```python
from build123d import *

# Parameters (mm, degrees)
SKETCH_1_W          = 55
SKETCH_1_H          = 20
SKETCH_1_R          = 4.5
EXTRUDE_1_DEPTH     = 20
EXTRUDE_START       = -10
EXTRUDE_2_OUTLINE_W = 13.25368731
EXTRUDE_2_OUTLINE_H = 35
EXTRUDE_2_DEPTH     = 20
SKETCH_3_R          = 5.25
CUT_EXTRUDE_1_DEPTH = 30
FILLET1_R           = 10
FILLET2_R           = 3
FILLET3_R           = 3


# Read off the part's stored shape, not the designer's step: 填料-伸長2
with BuildPart() as part:
    # 草圖1 → 填料-伸長1 (new body)
    with BuildSketch(Plane(origin=(0, 0, 0), x_dir=(1, 0, 0), z_dir=(0, 1, 0))):
        Rectangle(SKETCH_1_W, SKETCH_1_H)
        with Locations(Location((-15, 0, 0), (0, 0, 270))):
            Circle(SKETCH_1_R, mode=Mode.SUBTRACT)
        with Locations(Location((15, 0, 0), (0, 0, 90))):
            Circle(SKETCH_1_R, mode=Mode.SUBTRACT)
    extrude(amount=EXTRUDE_1_DEPTH)

    # 填料-伸長2 outline → 填料-伸長2 (add)
    with BuildSketch(Plane.XY.offset(EXTRUDE_START)):
        with Locations((0, 37.5)):
            Rectangle(EXTRUDE_2_OUTLINE_W, EXTRUDE_2_OUTLINE_H)
    extrude(amount=EXTRUDE_2_DEPTH)

    # 草圖3 → 除料-伸長1 (cut)
    with BuildSketch(Plane(origin=(6.626843655, 0, 0), x_dir=(0, 0, -1), z_dir=(1, 0, 0))):
        with Locations((0.362292653, 41.5)):
            Circle(SKETCH_3_R)
    extrude(amount=-CUT_EXTRUDE_1_DEPTH, mode=Mode.SUBTRACT)

    # Fillet1
    fillet1_edges = [part.edges().sort_by_distance(p)[0] for p in [
        (0, 55, -10),
        (0, 55, 10),
    ]]
    fillet(fillet1_edges, radius=FILLET1_R - 0.0001)  # a hair under: the kernel refuses the full size

    # Fillet2
    fillet2_edges = [part.edges().sort_by_distance(p)[0] for p in [
        (-27.5, 20, 0),
        (-17.063421827, 20, 10),
        (-17.063421827, 20, -10),
    ]]
    fillet(fillet2_edges, radius=FILLET2_R)

    # Fillet3
    fillet3_edges = [part.edges().sort_by_distance(p)[0] for p in [
        (17.063421827, 20, 10),
        (27.5, 20, 0),
        (17.063421828, 20, -10),
    ]]
    fillet(fillet3_edges, radius=FILLET3_R)


solid = part.part
```
Check sheet for the modelled part. Datum: model origin and axes. Units: mm. A direction names the side the tool comes from. Round coordinates to 2 decimals unless told otherwise and drop trailing zeros. Write each loop counter-clockwise with the first axis right and the second up, starting at its lowest first coordinate (ties: lowest second). Pieces come first, ordered by that corner, then holes. Notation, with made-up numbers: (-5, 29.25) -> (5, 29.25) arc R20 ccw to (5, 60.25) -> close; hole circle Ø10 at (63, -32.5). An arc over 180 degrees is marked (long way). One line per question, with ' | ' between items. Start each with the question number.
1. Release check for a two-part mould opening along Z. For faces 1 (the face through (0, 0, 0)), 2 (the face through (-10.54, 9.86, -0.59)), 3 (the face through (0.09, 51.99, -7.15)) record: +Z half, -Z half, draft (parallel to the pull), parting line (faces both ways), or undercut.
2. Sectioned sample at B-B, the plane y = 41.5. Record the cut outline in (x, z), then the cut area to 3 significant figures.
3. Sectioned sample at D-D, the plane y = 16. Record the cut outline in (x, z).
4. Sectioned sample at C-C, the plane x = -15. Record the cut outline in (y, z), then the cut area to 3 significant figures.
5. Scan lines: line 1 along X through (y, z) = (7.25, 0); line 2 along X through (y, z) = (16, 3.25); line 3 along Y through (x, z) = (11, 7.25). Record each from-to range of solid material in increasing order. Write a range as from..to.
6. Depth check by flat-ended pin: pin 1 (4 mm diameter, centred on x = 15.5, z = 2.5, fed in from +Y); pin 2 (10 mm diameter, centred on y = 35.5, z = 3.5, fed in from +X); pin 3 (4 mm diameter, centred on y = 28.5, z = 6, fed in from -X). Enter the tip coordinate at first touch or a pass-through.
7. Set-up check for faces 4 (the face through (-20, 20, 0)), 5 (the face through (-16.92, 19.1, 9.14)), 6 (the face through (17.21, 19.1, 9.14)), 7 (the face through (-16.92, 19.14, -9.1)): record each of +Z, -Z, +X, -X, +Y, -Y from which the full face is reachable in a straight line by a thin tool's end or side.
Taken from the geometry:
1) face 1: draft | face 2: undercut | face 3: -Z half
2) outline: (-6.63, -10) -> (6.63, -10) -> (6.63, -5.61) -> (-6.63, -5.61) -> close; (-6.63, 4.89) -> (6.63, 4.89) -> (6.63, 10) -> (-6.63, 10) -> close | area: 126 mm^2
3) outline: (-27.5, -10) -> (27.5, -10) -> (27.5, 10) -> (-27.5, 10) -> close; hole circle Ø9 at (-15, 0); hole circle Ø9 at (15, 0)
4) outline: (0, -10) -> (17, -10) arc R3 ccw to (20, -7) -> (20, -4.5) -> (0, -4.5) -> close; (0, 4.5) -> (20, 4.5) -> (20, 7) arc R3 ccw to (17, 10) -> (0, 10) -> close | area: 216 mm^2
5) line 1: x = -27.5..-19.5, -10.5..10.5, 19.5..27.5 | line 2: x = -27.5..-18.11, -11.89..11.89, 18.11..27.5 | line 3: y = 0..19.99
6) pin 1: stops at y = 20 | pin 2: stops at x = 6.63 | pin 3: stops at x = -6.63
7) face 4: +Z, -Z, -X, +Y | face 5: +Z, -X, +Y | face 6: +Z, +X, +Y | face 7: -Z, -X, +Y
